Can you work these out from the model? Positions are in its coordinate system, mm. A direction names the side the tool comes from. Coordinates: 2 decimals unless noted, no trailing zeros. Loops run counter-clockwise (first coordinate to the right, second up) from the corner with the lowest first, then second, coordinate; pieces in that order, holes last. Notation, with made-up numbers: M 46,3.25 L 102,3.25 A18 ccw 102,33.25 Z; hole C -6,-14 d10. An arc over 180 degrees is marked long. Return JSON: item names as keys, results as strings. Group by question number.
Autodesk Inventor part; units mm, degrees
ref_plane "YZ Plane" through (0, 0, 0) normal (1, 0, 0) x (0, 1, 0)
ref_plane "XZ Plane" through (0, 0, 0) normal (0, 1, 0) x (-1, 0, 0)
ref_plane "XY Plane" through (0, 0, 0) normal (0, 0, 1) x (1, 0, 0)
sketch "Sketch1" plane through (0, 0, 0) normal (0, 0, 1) x (1, 0, 0)
  arc A0 (1.8788, 9.9306) -> (-9.665, -8.9721) centre (-3.1084, 0) ccw
  arc A1 (287.3193, -140.2716) -> (281.1939, -130.341) centre (276.2068, -140.2716) ccw
  arc A2 (269.6501, -213.0916) -> (287.3193, -204.1195) centre (276.2068, -204.1195) ccw
  line L0 (1.8788, 9.9306) -> (281.1939, -130.341)
  line L1 (287.3193, -140.2716) -> (287.3193, -204.1195)
  line L2 (269.6501, -213.0916) -> (-9.665, -8.9721)
  arc A3 (3.3036, 12.7679) -> (-11.5383, -11.5355) centre (-3.1084, 0) ccw
  arc A4 (290.4943, -140.2716) -> (282.6188, -127.5037) centre (276.2068, -140.2716) ccw
  arc A5 (267.7768, -215.655) -> (290.4943, -204.1195) centre (276.2068, -204.1195) ccw
  line L3 (290.4943, -140.2716) -> (290.4943, -204.1195)
  line L4 (-11.5383, -11.5355) -> (267.7768, -215.655)
  line L5 (282.6188, -127.5037) -> (3.3036, 12.7679)
  point P0 (0, 0)
  dimension "d0" = 11.1125
  dimension "d1" = 3.175
extrude "Extrusion1" add sketch "Sketch1" along normal blind 10.16
properties part number "ShooterBelt" material "Rubber"
1) If I drill on line 1 (Y direction, x = 70, z = 3.25); line 2 (Y direction, x = 104.5, z = 4.5); line 3 (X direction, y = -131, z = 5.5), over which ranges is the centre line in solid material (lowest first)? Write a range as from..to.
2) For pin 1 (5 mm diameter, centred on x = 253.5, z = 7, fed in from +Y); pin 2 (2 mm diameter, centred on x = 67, z = 3, fed in from +Y); pin 3 (4 mm diameter, centred on y = -68.5, z = 1.5, fed in from -X), each with a flat end and sliding along its axis, tell me the tip position at first contact or that it passes through.
3) If we mould it in two halves opening along X, with no side actions, what happens to faces 3 (the face through (126.164, -112.166, 5.009)), 4 (the face through (290.494, -172, 5)), 5 (the face through (281.39, -213.95, 5.01))? For each: +X half, -X half, draft (parallel to the pull), parting line (faces both ways), or undercut.
4) For faces 1 (the face through (282.87, -216.76, 5.01)), 2 (the face through (131.95, -112.46, 5.01)), which set-ups out of +Z, -Z, +X, -X, +Y, -Y let a thin tool reach every point of the face, with its end or its side?
5) Suppose I cut it at C-C, the plane x = 21. List the corners of the cut face in (y, z) for me, then the cut area to 4 significant figures.
6) Suppose I cut it at B-B, the plane z = 7.5. List the corners of the cut face in (x, y) for me (1 decimal), then the cut area to 3 significant figures.
7) Suppose I cut it at A-A, the plane y = -134.5. List the corners of the cut face in (x, z) for me.
Returned:
{
 "1": {"line 1": "y = -71.12..-67.19, -24.28..-20.73", "line 2": "y = -96.33..-92.4, -41.61..-38.05", "line 3": "x = 151.94..157.32, 282.33..287.08"},
 "2": {"pin 1": "stops at y = -111.62", "pin 2": "stops at y = -18.72", "pin 3": "stops at x = 63.67"},
 "3": {"face 3": "-X half", "face 4": "+X half", "face 5": "undercut"},
 "4": {"face 1": "+Z, -Z, -Y", "face 2": "+Z, -Z"},
 "5": {"outline": "M -35.31,0 L -31.38,0 L -31.38,10.16 L -35.31,10.16 Z; M 0.33,0 L 3.88,0 L 3.88,10.16 L 0.33,10.16 Z", "area": "76.05 mm²"},
 "6": {"outline": "M -11.5,-11.5 L 267.8,-215.7 A14.3 ccw 290.5,-204.1 L 290.5,-140.3 A14.3 ccw 282.6,-127.5 L 3.3,12.8 A14.3 ccw Z; hole M -9.7,-9 L 269.7,-213.1 A11.1 ccw 287.3,-204.1 L 287.3,-140.3 A11.1 ccw 281.2,-130.3 L 1.9,9.9 A11.1 ccw Z", "area": "2,550 mm²"},
 "7": {"outline": "M 156.73,0 L 162.11,0 L 162.11,10.16 L 156.73,10.16 Z; M 285.7,0 L 289.28,0 L 289.28,10.16 L 285.7,10.16 Z"}
}
